from build123d import *

# Parameters (mm, degrees)
BOSS_EXTRUDE1_DEPTH = 4.75
FILLET2_R           = 0.2
FILLET3_R           = 1
FILLET5_R           = 0.5
FILLET6_R           = 1
SKETCH3_W           = 6.37
SKETCH3_H           = 4.75
BOSS_EXTRUDE2_DEPTH = 2
SKETCH4_W           = 6.5
SKETCH4_H           = 6.5
BOSS_EXTRUDE3_DEPTH = 3
SKETCH5_W           = 4.6
SKETCH5_H           = 0.5
CUT_EXTRUDE1_DEPTH  = 6
SKETCH8_W           = 4
SKETCH8_H           = 4
CUT_EXTRUDE2_DEPTH  = 0.5
SKETCH9_R           = 1.7145
BOSS_EXTRUDE4_DEPTH = 12.668


with BuildPart() as part:
    # Sketch2 → Boss-Extrude1 (new body)
    with BuildSketch(Plane(origin=(0, 0, 0), x_dir=(1, 0, 0), z_dir=(0, 1, 0))):
        Polygon((-3.269672992, 3.380584559), (-3.269672992, 7.934769302), (-3.769672992, 7.934769302), (-3.269672992, 8.862323318), (-1.769672992, 8.862323318), (-1.769672992, 3.380584559), (-1.769672992, -0.429415441), (2.600327008, -0.429415441), (2.600327008, 3.380584559), (2.600327008, 8.862323318), (4.100327008, 8.862323318), (4.600327008, 7.934769302), (4.100327008, 7.934769302), (4.100327008, 5.316430627), (4.100327008, -4.239415441), (-3.269672992, -4.239415441), align=None)
    extrude(amount=BOSS_EXTRUDE1_DEPTH)

    # Fillet2
    fillet2_edges = [part.edges().sort_by_distance(p)[0] for p in [
        (-3.769672992, 2.375, -7.934769302),
        (4.600327008, 2.375, -7.934769302),
    ]]
    fillet(fillet2_edges, radius=FILLET2_R)

    # Fillet3
    # the kernel refuses this fillet: 1 mm, written as the material it takes off along each edge
    with BuildSketch(Plane(origin=(-1.769672992, -2.5, -8.862323318), x_dir=(-1, 0, 0), z_dir=(0, 1, 0)), Plane(origin=(2.600327008, -2.5, -8.862323318), x_dir=(0, 0, 1), z_dir=(0, 1, 0))) as fillet3_piece_1:
        with BuildLine():
            CenterArc((FILLET3_R, FILLET3_R), FILLET3_R, 180, 90)
            Line((0, FILLET3_R), (0, 0))
            Line((0, 0), (FILLET3_R, 0))
        make_face()
    extrude(amount=9.75, mode=Mode.SUBTRACT)
    with BuildSketch(Plane(origin=(4.100327008, -1.492458976, -8.862323318), x_dir=(0.47450281579704723, 0, 0.8802539848252171), z_dir=(0, 1, 0))) as fillet3_piece_2:
        with BuildLine():
            CenterArc((FILLET3_R * 0.596983590262, -FILLET3_R), FILLET3_R, 90, 61.673016648)
            Line((-FILLET3_R * 0.283270394564, -FILLET3_R * 0.525497184203), (0, 0))
            Line((0, 0), (FILLET3_R * 0.596983590262, 0))
        make_face()
    extrude(amount=7.734917951, mode=Mode.SUBTRACT)
    with BuildSketch(Plane(origin=(-3.269672992, -1.492458976, -8.862323318), x_dir=(-0.474502815797046, 0, 0.8802539848252178), z_dir=(0, 1, 0))) as fillet3_piece_3:
        with BuildLine():
            CenterArc((FILLET3_R * 0.596983590262, FILLET3_R), FILLET3_R, 208.326983352, 61.673016648)
            Line((-FILLET3_R * 0.283270394564, FILLET3_R * 0.525497184203), (0, 0))
            Line((0, 0), (FILLET3_R * 0.596983590262, 0))
        make_face()
    extrude(amount=7.734917951, mode=Mode.SUBTRACT)

    # Fillet5
    fillet5_edges = [part.edges().sort_by_distance(p)[0] for p in [
        (-3.269672992, 0, -1.84767693),
        (4.100327008, 0, -1.84767693),
        (4.100327008, 4.75, -1.84767693),
        (-3.269672992, 4.75, -1.84767693),
    ]]
    fillet(fillet5_edges, radius=FILLET5_R)

    # Fillet6
    fillet6_edges = [part.edges().sort_by_distance(p)[0] for p in [
        (-1.769672992, 2.375, 0.429415441),
        (2.600327008, 2.375, 0.429415441),
    ]]
    fillet(fillet6_edges, radius=FILLET6_R)

    # Sketch3 → Boss-Extrude2 (add)
    with BuildSketch(Plane.XY.offset(4.239415441)):
        with Locations((0.415327008, 2.375)):
            Rectangle(SKETCH3_W, SKETCH3_H)
    extrude(amount=BOSS_EXTRUDE2_DEPTH)

    # Sketch4 → Boss-Extrude3 (add)
    with BuildSketch(Plane.XY.offset(6.239415441)):
        with Locations((0.415327008, 2.375)):
            Rectangle(SKETCH4_W, SKETCH4_H)
    extrude(amount=BOSS_EXTRUDE3_DEPTH)

    # Sketch5 → Cut-Extrude1 (cut)
    with BuildSketch(Plane(origin=(0, 5.625, 0), x_dir=(1, 0, 0), z_dir=(0, 1, 0))):
        with Locations((0.415327008, -8.589415441)):
            Rectangle(SKETCH5_W, SKETCH5_H)
    extrude(amount=-CUT_EXTRUDE1_DEPTH, mode=Mode.SUBTRACT)

    # Sketch8 → Cut-Extrude2 (cut)
    with BuildSketch(Plane.XY.offset(9.239415441)):
        with Locations((0.415327008, 2.375)):
            Rectangle(SKETCH8_W, SKETCH8_H)
    extrude(amount=-CUT_EXTRUDE2_DEPTH, mode=Mode.SUBTRACT)

    # Sketch9 → Boss-Extrude4 (add)
    with BuildSketch(Plane(origin=(0, 0, 0.429415441), x_dir=(-1, 0, 0), z_dir=(0, 0, -1))):
        with Locations(Location((-0.415327008, 2.375, 0), (0, 0, 133.722288973))):
            Circle(SKETCH9_R)
    extrude(amount=BOSS_EXTRUDE4_DEPTH)


solid = part.part
Design review of the part built by this model. Coordinates are the model's own, in mm. A direction names the side the tool comes from. Coordinates: 2 decimals unless noted, no trailing zeros. Order: outer loops, then holes, each group sorted by start corner. A loop starts at its lowest first (then second) coordinate and runs counter-clockwise, first axis right, second up. Notation, with made-up numbers: (-28.5, 35) - (15.5, 35) arc R38 cw to (15.5, 73) - close; hole circle Ø8 at (61.5, -31.75). An arc over 180 degrees is marked (long way). Put each result on its own line as item: value.
1) Wall thickness on L1, parallel to X at y = 2.5, z = -7; L2, parallel to Z at x = 1.5, y = 5; L3, parallel to Z at x = 0, y = 0.25: over which ranges is each line inside the solid? List them lowest first. Write a range as from..to.
Response values:
L1: x = -3.27..-1.77, -1.29..2.13, 2.6..4.1
L2: z = 6.24..8.34, 8.84..9.24
L3: z = 0.43..8.34, 8.84..9.24
2) Insertion check: P1, Ø1.4, axis at x = 1.5, y = 3.5, coming from the +Z side; P2, Ø1.5, axis at x = -1.5, z = 2, coming from the -Y side; P3, Ø2, axis at y = 3.5, z = -5.5, coming from the -X side. Each pin has a flat end and moves straight along its axis. Give the tip position at first contact, or say it passes through.
Response values:
P1: stops at z = 8.34
P2: stops at y = 0
P3: stops at x = -3.27
3) Take a section at D-D, the plane x = 3.25. Give the boundary of the cut face in (y, z) (3 decimals).
Response values:
outline: (-0.875, 6.239) - (0, 6.239) - (0, -8.799) - (4.75, -8.799) - (4.75, 6.239) - (5.625, 6.239) - (5.625, 9.239) - (-0.875, 9.239) - close
4) Tool access review of faces 1 (the face through (-3.27, 2, -2)), 2 (the face through (0, 5, 8.839)), 3 (the face through (0, 4.75, 2)): name each direction out of +Z, -Z, +X, -X, +Y, -Y from which nothing blocks a thin tool from reaching the whole face with its end or side.
Response values:
face 1: +Z, -X, +Y, -Y
face 2: +Y
face 3: -Z, +X, -X, +Y
5) Take a section at B-B, the plane x = -0.5. Give the boundary of the cut face in (y, z) (3 decimals), and give its area (3 significant figures).
Response values:
outline: (-0.875, 6.239) - (0, 6.239) - (0, 0.429) - (0.925, 0.429) - (0.925, -12.239) - (3.825, -12.239) - (3.825, 0.429) - (4.75, 0.429) - (4.75, 6.239) - (5.625, 6.239) - (5.625, 8.339) - (-0.375, 8.339) - (-0.375, 8.839) - (0.375, 8.839) - (0.375, 9.239) - (-0.875, 9.239) - close; (4.375, 8.839) - (5.625, 8.839) - (5.625, 9.239) - (4.375, 9.239) - close
area: 79.2 mm²
6) Take a section at A-A, the plane z = -5. Count the separate pieces of the cut face and the enclosed holes in it, and give its area (3 significant figures).
Response values:
separate pieces: 3
enclosed holes: 0
area: 23.3 mm²
7) The part is to be moulded in two halves that separate along Z. For faces 4 (the face through (2.6, 2, -4)), 5 (the face through (0, 2, -12.239)), 6 (the face through (0, 3, 8.339)), say which applies: released by +Z, released by -Z, zero draft, split by the parting line, or undercut.
Response values:
face 4: zero draft
face 5: released by -Z
face 6: undercut
8) Take a section at C-C, the plane z = 2. Give the boundary of the cut face in (x, y), and give its area (3 significant figures).
Response values:
outline: (-3.27, 0.5) arc R0.5 ccw to (-2.77, 0) - (3.6, 0) arc R0.5 ccw to (4.1, 0.5) - (4.1, 4.25) arc R0.5 ccw to (3.6, 4.75) - (-2.77, 4.75) arc R0.5 ccw to (-3.27, 4.25) - close
area: 34.8 mm²
